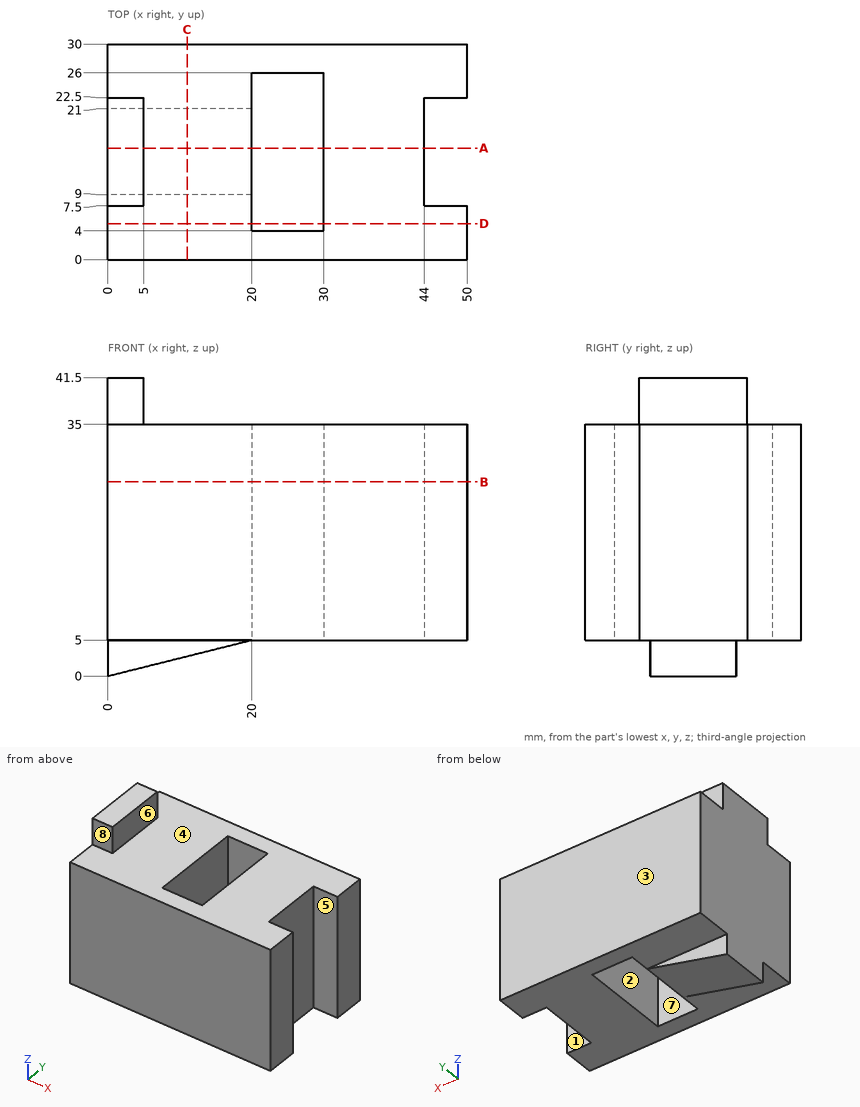
Study the drawing (mm; zero at the part's minimum x, y, z) and answer. A direction names the side the tool comes from. Give positions to 0.01 mm unless a question says otherwise; leave off trailing zeros. Write each loop counter-clockwise with the first axis right and the second up, starting at its lowest first coordinate (ties: lowest second). Pieces come first, ordered by that corner, then holes. Notation, with made-up numbers: (-26, 67.5) - (0, 67.5) arc R9 ccw to (0, 76.5) - close; hole circle Ø9 at (-13, 4.5). An arc over 180 degrees is marked (long way). Use CSV: the item, a comma, the result in double quotes. Start each with the question number.
(1) Find section B-B (z = 27). Give the vertices of the cut face in (x, y).
(2) For the marked faces 5, 6, 7 and 8, determine the directions among +Z, -Z, +X, -X, +Y, -Y from which every point of the face is accessible in a straight line to the end or side of a thin tool.
(3) Determine the mould class of the marked faces 1, 2, 3 and 4 for opening direction Y: +Y half, -Y half, draft (parallel to the pull), parting line (faces both ways), or undercut.
(4) Find section C-C (x = 11). Give the vertices of the cut face in (y, z).
(5) Find section A-A (y = 15.5). Give the vertices of the cut face in (x, z).
(6) Consider line 1 along Y through (x, z) = (48, 20.5); line 2 along X through (y, z) = (13.5, 33.5); line 3 along X through (y, z) = (6.75, 33). Determine where each line is inside the solid, lowest interval first.
(7) Given P1, Ø5, axis at x = 6.5, y = 8.5, coming from the -Z side; P2, Ø5.5, axis at x = 11.5, z = 1.5, coming from the +Y side; P3, Ø4, axis at x = 14, z = 2, coming from the -Y side, each flat-ended and moving along its own axis, determine where each tip first touches the part or whether it passes through.
(8) Find section D-D (y = 5). Give the vertices of the cut face in (x, z).
Findings below:
1,outline,"(0, 0) - (50, 0) - (50, 7.5) - (44, 7.5) - (44, 22.5) - (50, 22.5) - (50, 30) - (0, 30) - close; hole (20, 4) - (30, 4) - (30, 26) - (20, 26) - close"
2,face 5,"+Z, -Z, +X"
2,face 6,"+Z, +X, +Y, -Y"
2,face 7,"+Z, -Z"
2,face 8,"+Z, +X, -X, -Y"
3,face 1,"undercut"
3,face 2,"undercut"
3,face 3,"+Y half"
3,face 4,"draft"
4,outline,"(0, 5) - (9, 5) - (9, 2.75) - (21, 2.75) - (21, 5) - (30, 5) - (30, 35) - (0, 35) - close"
5,outline,"(0, 0) - (20, 5) - (20, 35) - (5, 35) - (5, 41.5) - (0, 41.5) - close; (30, 5) - (44, 5) - (44, 35) - (30, 35) - close"
6,line 1,"0 to 7.5, 22.5 to 30"
6,line 2,"0 to 20, 30 to 44"
6,line 3,"0 to 20, 30 to 50"
7,P1,"z = 1.01"
7,P2,"y = 21"
7,P3,"y = 9"
8,outline,"(0, 5) - (20, 5) - (20, 35) - (0, 35) - close; (30, 5) - (50, 5) - (50, 35) - (30, 35) - close"
